Geometry: final body of the model. Coordinates: model frame, mm. A direction names the side the tool comes from. Round coordinates to 2 decimals unless told otherwise and drop trailing zeros. Loops run counter-clockwise (first coordinate to the right, second up) from the corner with the lowest first, then second, coordinate; pieces in that order, holes last. Notation, with made-up numbers: (40, 44.25) - (84, 44.25) arc R16 cw to (84, 74.25) - close; hole circle Ø6 at (-35, -37.75). An arc over 180 degrees is marked (long way). Answer as a JSON object with one key per item and string values. Group by question number.
Item 1: Section B-B (x = -9.5). Return the cut outline in (y, z).
Item 2: Line query: line 1 (X direction, y = 36, z = -27.5); line 2 (Y direction, x = -14.5, z = 158.5); line 3 (Y direction, x = -1, z = 95). Output: solid intervals per line, ascending.
Item 3: Reachability of faces 1 (the face through (-20, 20, 6)), 2 (the face through (-10, 38.5, 6)) from +Z, -Z, +X, -X, +Y, -Y: full face, straight path, thin tool, end or side. Return the list, or none.
Item 4: Draft query along Y for faces 3 (the face through (-10, 1.5, 6)), 4 (the face through (-19, 22, -430)), 5 (the face through (-10, 40, 6)), 6 (the face through (-18.5, 20, 6)). Return one class per face: released by +Y, released by -Y, zero draft, split by the parting line, or undercut.
Item 5: Section A-A (y = 16.5). Return the cut outline in (x, z), plus the area to 3 significant figures.
Item 6: Section C-C (z = -75). Return the cut outline in (x, y).
```python
from build123d import *

# Parameters (mm, degrees)
EXTRUDE_1_DEPTH = 430


# Read off the part's stored shape, not the designer's step: Бобышка-Вытянуть1
with BuildPart() as part:
    # Бобышка-Вытянуть1 outline → Бобышка-Вытянуть1 (new body)
    with BuildSketch(Plane.XY):
        with BuildLine():
            Line((0, 1.5), (0, 38.5))
            ThreePointArc((0, 38.5), (-0.439339828, 39.560660172), (-1.5, 40))
            Line((-1.5, 40), (-18.5, 40))
            ThreePointArc((-18.5, 40), (-19.560660172, 39.560660172), (-20, 38.5))
            Line((-20, 38.5), (-20, 1.5))
            ThreePointArc((-20, 1.5), (-19.560660172, 0.439339828), (-18.5, 0))
            Line((-18.5, 0), (-1.5, 0))
            ThreePointArc((-1.5, 0), (-0.439339828, 0.439339828), (0, 1.5))
        make_face()
        with BuildLine():
            ThreePointArc((-1.5, 2.5), (-1.792893219, 1.792893219), (-2.5, 1.5))
            Line((-2.5, 1.5), (-17.5, 1.5))
            ThreePointArc((-17.5, 1.5), (-18.207106781, 1.792893219), (-18.5, 2.5))
            Line((-18.5, 2.5), (-18.5, 37.5))
            ThreePointArc((-18.5, 37.5), (-18.207106781, 38.207106781), (-17.5, 38.5))
            Line((-17.5, 38.5), (-2.5, 38.5))
            ThreePointArc((-2.5, 38.5), (-1.792893219, 38.207106781), (-1.5, 37.5))
            Line((-1.5, 37.5), (-1.5, 2.5))
        make_face(mode=Mode.SUBTRACT)
    extrude(amount=EXTRUDE_1_DEPTH)

    # Зеркальное отражение1: part across plane


with BuildPart() as part_1:
    add(part.part)
    add(part.part.mirror(Plane(origin=(-1.5, 38.5, 0), x_dir=(1, 0, 0), z_dir=(0, 0, -1))))


solid = part_1.part
```
Values:
{
 "1": {"outline": "(0, -430) - (1.5, -430) - (1.5, 430) - (0, 430) - close; (38.5, -430) - (40, -430) - (40, 430) - (38.5, 430) - close"},
 "2": {"line 1": "x = -20 to -18.5, -1.5 to 0", "line 2": "y = 0 to 1.5, 38.5 to 40", "line 3": "y = 0.09 to 39.91"},
 "3": {"face 1": "+Z, -Z, -X, +Y, -Y", "face 2": "+Z, -Z"},
 "4": {"face 3": "undercut", "face 4": "zero draft", "face 5": "released by +Y", "face 6": "undercut"},
 "5": {"outline": "(-20, -430) - (-18.5, -430) - (-18.5, 430) - (-20, 430) - close; (-1.5, -430) - (0, -430) - (0, 430) - (-1.5, 430) - close", "area": "2,580 mm^2"},
 "6": {"outline": "(-20, 1.5) arc R1.5 ccw to (-18.5, 0) - (-1.5, 0) arc R1.5 ccw to (0, 1.5) - (0, 38.5) arc R1.5 ccw to (-1.5, 40) - (-18.5, 40) arc R1.5 ccw to (-20, 38.5) - close; hole (-18.5, 2.5) arc R1 ccw to (-17.5, 1.5) - (-2.5, 1.5) arc R1 ccw to (-1.5, 2.5) - (-1.5, 37.5) arc R1 ccw to (-2.5, 38.5) - (-17.5, 38.5) arc R1 ccw to (-18.5, 37.5) - close"}
}
